Can you work these out from the model? Positions are in its coordinate system, mm. Give positions to 0.01 mm unless a question says otherwise; leave off trailing zeros. Write each loop counter-clockwise with the first axis right and the second up, starting at its lowest first coordinate (ties: lowest second). Pieces come first, ordered by that corner, then holes.
```python
from build123d import *

# Parameters (mm, degrees)
PAD_DEPTH   = 20
SKETCH002_R = 10


with BuildPart() as part:
    # Sketch → Pad (new body)
    with BuildSketch(Plane.XY):
        Polygon((100, 0), (50, 86.60254), (-50, 86.60254), (-100, 0), (-50, -86.60254), (50, -86.60254), align=None)
    extrude(amount=PAD_DEPTH)

    # Sketch001 → Revolution (revolve)
    with BuildSketch(Plane.XZ):
        with BuildLine():
            ThreePointArc((-25, 55), (-24.74611, 37.179127), (-20, 20))
            Line((-20, 20), (-18, 20))
            ThreePointArc((-23, 55), (-22.74611, 37.179127), (-18, 20))
            Line((-25, 55), (-23, 55))
        make_face()
    revolve(axis=Axis((0, 0, 0), (0, 0, 1)))

    # Sketch002 → Groove (revolve, cut)
    with BuildSketch(Plane.XZ):
        with Locations((35, 20)):
            Circle(SKETCH002_R)
    revolve(axis=Axis((0, 0, 0), (0, 0, 1)), mode=Mode.SUBTRACT)


solid = part.part
```
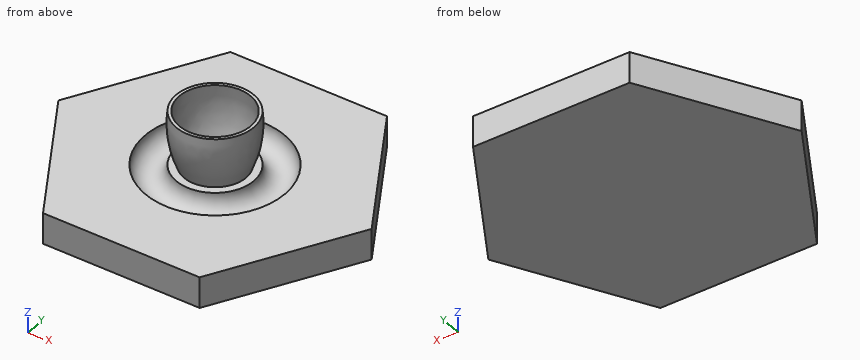
1) Suppose I cut it at B-B on z = 7. Write out the boundary of the cut face in (x, y).
Values follow:
outline: (-100, 0) - (-50, -86.6) - (50, -86.6) - (100, 0) - (50, 86.6) - (-50, 86.6) - close
2) For pin 1 Ø12 at (x, y) = (3.5, 31) entering from -Z; pin 2 Ø5 at (y, z) = (0, 43) entering from -X, each with a flat end and sliding along its axis, tell me the tip position at first contact or that it passes through.
Values follow:
pin 1: stops at z = 0
pin 2: stops at x = -25.43
3) Please list where these lines run through material, in increasing order: L1, parallel to Y at x = -9, z = 16; L2, parallel to X at y = 13, z = 19; L3, parallel to Z at x = 41, y = 51.
Values follow:
L1: y = -86.6 to -43.24, -24.22 to 24.22, 43.24 to 86.6
L2: x = -92.49 to -43.03, -21.41 to 21.41, 43.03 to 92.49
L3: z = 0 to 20
4) Suppose I cut it at C-C on y = -53. Write out the boundary of the cut face in (x, z).
Values follow:
outline: (-69.4, 0) - (69.4, 0) - (69.4, 20) - (-69.4, 20) - close
5) Suppose I cut it at D-D on x = 71.5. Write out the boundary of the cut face in (y, z), plus the area to 3 significant figures.
Values follow:
outline: (-49.36, 0) - (49.36, 0) - (49.36, 20) - (-49.36, 20) - close
area: 1,970 mm2
6) Suppose I cut it at A-A on z = 17. Write out the boundary of the cut face in (x, y).
Values follow:
outline: (-100, 0) - (-50, -86.6) - (50, -86.6) - (100, 0) - (50, 86.6) - (-50, 86.6) - close; circle Ø50.92 at (0, 0); hole circle Ø89.08 at (0, 0)
